from build123d import *

# Parameters (mm, degrees)
F1_DEPTH = 30
F2_R     = 13
F3_DEPTH = 15
F5_DEPTH = 15
F6_W     = 16.029888
F6_H     = 19.464858
F7_DEPTH = 10
F8_R     = 10


with BuildPart() as f1:
    # F0 (on Right) → F1 (new body)
    with BuildSketch(Plane.YZ):
        with BuildLine():
            ThreePointArc((69.107138, 0), (34.553569, -34.553569), (0, 0))
            Line((0, 0), (0, 150))
            Line((0, 150), (-30, 150))
            Line((-30, 150), (-30, 0))
            ThreePointArc((-30, 0), (34.553569, -64.553569), (99.107138, 0))
            ThreePointArc((99.107138, 0), (84.107138, 14.337759), (69.107138, 0))
        make_face()
    extrude(amount=F1_DEPTH)

    # F2 (on face) → F3 (cut)
    with BuildSketch(Plane.YZ.offset(30)):
        with Locations((-15, 95.836063)):
            Circle(F2_R)
    extrude(amount=-F3_DEPTH, mode=Mode.SUBTRACT)

    # F4 (on face) → F5 (cut)
    with BuildSketch(Plane.XZ.offset(30)):
        with BuildLine():
            Line((13, 130.011459), (13, 125.511459))
            ThreePointArc((13, 125.511459), (15, 118.047357), (17, 125.511459))
            Line((17, 125.511459), (17, 130.011459))
            ThreePointArc((17, 130.011459), (15, 132.011459), (13, 130.011459))
        make_face()
    extrude(amount=-F5_DEPTH, mode=Mode.SUBTRACT)

    # F6 (on face) → F7 (cut)
    with BuildSketch(Plane.XZ.offset(15)):
        with Locations((15.266558, 124.901053)):
            Rectangle(F6_W, F6_H)
    extrude(amount=F7_DEPTH, mode=Mode.SUBTRACT)

    # F8
    f8_edges = [f1.edges().sort_by_distance(p)[0] for p in [
        (15, 0, 150),
        (15, -30, 150),
    ]]
    fillet(f8_edges, radius=F8_R)


solid = f1.part
CAD build for the part. Positions are in the model's coordinates, mm. A direction names the side the tool comes from. Round coordinates to 2 decimals unless told otherwise and drop trailing zeros. Order: outer loops, then holes, each group sorted by start corner. A loop starts at its lowest first (then second) coordinate and runs counter-clockwise, first axis right, second up. Notation, with made-up numbers: (27, 27.25) - (31, 27.25) arc R20 ccw to (31, 64.25) - close; hole circle Ø6 at (-30.5, -25). An arc over 180 degrees is marked (long way). Return JSON: item names as keys, results as strings.
(1) Cut at C-C (y = 74.5). Give the cut face in (x, z), then the cut area to 3 significant figures.
Answer key:
{"outline": "(0, -50.71) - (30, -50.71) - (30, 10.86) - (0, 10.86) - close", "area": "1,850 mm^2"}
(2) Wall check: probe 1 along Y at (x, z) = (19, 77); probe 2 along Y at (x, z) = (18.5, -2.5); probe 3 along Y at (x, z) = (13.75, -17). Give the ranges that are in metal, low to high. Write a range as from..to.
Answer key:
{"probe 1": "y = -30..0", "probe 2": "y = -29.95..0.09, 69.02..99.06", "probe 3": "y = -27.72..4.47, 64.64..96.83"}
(3) Pull direction Z, two halves, no side cores. Call faces 1 (the face through (15, -30, 71)), 2 (the face through (15.04, -27.54, 132.01)), 3 (the face through (14.79, 35.313, -34.545)): +Z half, -Z half, draft (parallel to the pull), parting line (faces both ways), or undercut.
Answer key:
{"face 1": "draft", "face 2": "undercut", "face 3": "+Z half"}
(4) Cut at B-B (z = 111). Give the cut face in (x, y).
Answer key:
{"outline": "(0, -30) - (30, -30) - (30, 0) - (0, 0) - close"}
(5) Tool access for faces 4 (the face through (15, -20, 134.633)), 5 (the face through (15.21, -2.85, 146.99)), 6 (the face through (14.85, -27.54, 118.05)), 7 (the face through (14.79, 84.428, 14.334)), 8 (the face through (22.605, -16.692, 108.725)): list every direction of +Z, -Z, +X, -X, +Y, -Y with a clear straight run to the whole face (end or side of a thin tool).
Answer key:
{"face 4": "none", "face 5": "+Z, +X, -X, +Y", "face 6": "-Y", "face 7": "+Z, +X, -X", "face 8": "+X"}
(6) Cut at A-A (x = 2.75). Give the cut face in (y, z).
Answer key:
{"outline": "(-30, 0) arc R64.55 ccw to (99.11, 0) arc R15.02 ccw to (69.11, 0) arc R34.55 cw to (0, 0) - (0, 140) arc R10 ccw to (-10, 150) - (-20, 150) arc R10 ccw to (-30, 140) - close"}
(7) Pin check, flat tips, straight feed: pin 1 Ø10 at (x, y) = (9, -14) entering from -Z; pin 2 Ø6 at (x, y) = (10, 37.5) entering from -Z; pin 3 Ø1.5 at (x, y) = (3, 12.5) entering from -Z. Stop position of each tip, or through.
Answer key:
{"pin 1": "stops at z = -47.65", "pin 2": "stops at z = -64.55", "pin 3": "stops at z = -60.94"}
